The model under review builds one solid part; all positions refer to its coordinate system, in mm. Face numbers are marked on the shaded views. A direction names the side the tool comes from. Coordinates: 2 decimals unless noted, no trailing zeros. Loops run counter-clockwise (first coordinate to the right, second up) from the corner with the lowest first, then second, coordinate; pieces in that order, holes last. Notation, with made-up numbers: M 22.25,-4.5 L 51.25,-4.5 A19 cw 51.25,23.5 Z; hole C -39.75,-24 d2. An arc over 180 degrees is marked long. Use CSV: the item, a comma, the result in double quotes. Start each with the question number.
1. Clearance check with flat-ended pins moving along their axes: P1, Ø5, axis at y = -18, z = -9.5, coming from the -X side; P2, Ø1, axis at y = 34, z = 2, coming from the -X side; P3, Ø12, axis at x = -8.5, y = -24, coming from the -Z side. State where each tip first meets the part, or that it passes through.
2. Tool access review of the marked faces 5, 6, 7, 8 and 9: name each direction out of +Z, -Z, +X, -X, +Y, -Y from which nothing blocks a thin tool from reaching the whole face with its end or side.
3. Add section D-D, the plane z = -14. Write out the cut boundary in (x, y), then the cut area to 3 significant figures.
4. Draft analysis for pull direction X (two halves, no side actions). For the marked faces 1, 2, 3 and 4, state which applies: +X half, -X half, draft (parallel to the pull), parting line (faces both ways), or undercut.
5. For L1, parallel to Y at x = 113.5, z = 0; L2, parallel to X at y = -11, z = 15; L3, parallel to X at y = -2.5, z = 0.5 (3 decimals), list the stretches that pass through material, from the lowest coordinate up.
6. Add section B-B, the plane z = 0. Write out the cut boundary in (x, y), then the cut area to 3 significant figures.
7. Add section C-C, the plane x = 106.5. Write out the cut boundary in (y, z).
8. Add section A-A, the plane y = 0. Write out the cut boundary in (x, z), then the cut area to 3 significant figures.
from build123d import *

# Parameters (mm, degrees)
SKETCH1_R           = 25
BOSS_EXTRUDE1_DEPTH = 50
SKETCH2_R           = 20
BOSS_EXTRUDE2_DEPTH = 30
SKETCH3_W           = 16.960857005
SKETCH3_H           = 10
BOSS_EXTRUDE3_DEPTH = 120
SKETCH4_W           = 20
SKETCH4_H           = 16.960857005
BOSS_EXTRUDE4_DEPTH = 50
SKETCH5_W           = 20
SKETCH5_H           = 20
BOSS_EXTRUDE5_DEPTH = 20
SKETCH6_R           = 3
CUT_EXTRUDE1_DEPTH  = 20


with BuildPart() as part:
    # Sketch1 → Boss-Extrude1 (new, symmetric)
    with BuildSketch(Plane(origin=(0, 0, 0), x_dir=(1, 0, 0), z_dir=(0, 1, 0))):
        with Locations(Location((0, 0, 0), (0, 0, 270))):
            Circle(SKETCH1_R)
    extrude(amount=BOSS_EXTRUDE1_DEPTH, both=True)

    # Sketch2 → Boss-Extrude2 (add)
    with BuildSketch(Plane(origin=(0, 0, 0), x_dir=(0, 0, -1), z_dir=(1, 0, 0))):
        with Locations(Location((0, 0, 0), (0, 0, 180))):
            Circle(SKETCH2_R)
    extrude(amount=BOSS_EXTRUDE2_DEPTH)

    # Sketch3 → Boss-Extrude3 (add)
    with BuildSketch(Plane(origin=(0, 0, 0), x_dir=(0, 0, -1), z_dir=(1, 0, 0))):
        with Locations((-16.519571497, 45)):
            Rectangle(SKETCH3_W, SKETCH3_H)
    extrude(amount=BOSS_EXTRUDE3_DEPTH)

    # Sketch4 → Boss-Extrude4 (add)
    with BuildSketch(Plane.XZ.offset(-40)):
        with Locations((110, 16.519571497)):
            Rectangle(SKETCH4_W, SKETCH4_H)
    extrude(amount=BOSS_EXTRUDE4_DEPTH)

    # Sketch5 → Boss-Extrude5 (add)
    with BuildSketch(Plane(origin=(0, 0, 8.039142995), x_dir=(-1, 0, 0), z_dir=(0, 0, -1))):
        with Locations((-110, 0)):
            Rectangle(SKETCH5_W, SKETCH5_H)
    extrude(amount=BOSS_EXTRUDE5_DEPTH)

    # Sketch6 → Cut-Extrude1 (cut)
    with BuildSketch(Plane(origin=(120, 0, 0), x_dir=(0, 0, -1), z_dir=(1, 0, 0))):
        Circle(SKETCH6_R)
    extrude(amount=-CUT_EXTRUDE1_DEPTH, mode=Mode.SUBTRACT)


solid = part.part
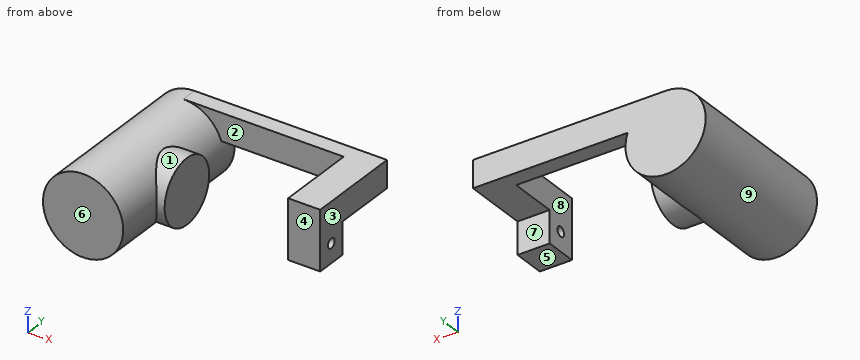
Computed:
1,P1,"stops at x = -24"
1,P2,"stops at x = -24.95"
1,P3,"stops at z = -24.87"
2,face 5,"-Z, +X, +Y, -Y"
2,face 6,"+Z, -Z, +X, -X, -Y"
2,face 7,"-Z, +X, +Y"
2,face 8,"+Z, -Z, -Y"
2,face 9,"none"
3,outline,"M -20.71,-50 L 20.71,-50 L 20.71,-14.28 L 30,-14.28 L 30,14.28 L 20.71,14.28 L 20.71,50 L -20.71,50 Z"
3,area,"4,410 mm^2"
4,face 1,"undercut"
4,face 2,"undercut"
4,face 3,"+X half"
4,face 4,"draft"
5,L1,"y = -10 to -3, 3 to 10"
5,L2,"x = -20 to 30"
5,L3,"x = -24.995 to 30"
6,outline,"M -25,-50 L 25,-50 L 25,-20 L 30,-20 L 30,20 L 25,20 L 25,50 L -25,50 Z; M 100,-10 L 120,-10 L 120,-3 L 100,-3 Z; M 100,3 L 120,3 L 120,10 L 100,10 Z"
6,area,"5,480 mm^2"
7,outline,"M -10,-11.96 L 10,-11.96 L 10,8.04 L 50,8.04 L 50,25 L -10,25 Z; hole C 0,0 d6"
8,outline,"M 15,-20 L 30,-20 L 30,20 L 15,20 A25 ccw long Z; M 100,-11.96 L 120,-11.96 L 120,-3 L 100,-3 Z; M 100,3 L 120,3 L 120,25 L 100,25 Z"
8,area,"2,900 mm^2"
